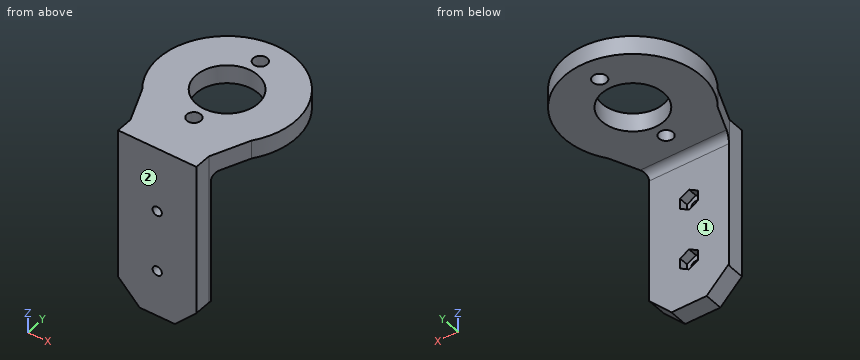
Autodesk Inventor part; units mm, degrees
ref_plane "YZ Plane" through (0, 0, 0) normal (1, 0, 0) x (0, 1, 0)
ref_plane "XZ Plane" through (0, 0, 0) normal (0, 1, 0) x (-1, 0, 0)
ref_plane "XY Plane" through (0, 0, 0) normal (0, 0, 1) x (1, 0, 0)
sketch "Sketch1" plane through (0, 0, 0) normal (0, 0, 1) x (1, 0, 0)
  circle A0 centre (0, 0) radius 22.1
  circle A1 centre (0, 14.5) radius 2.25
  circle A2 centre (0, -14.5) radius 2.25
  line L0 (0, 14.5) -> (0, -14.5)
  circle A3 centre (0, 0) radius 10
  line L1 (-12.7, -18.086459) -> (-12.7, -30.5)
  line L2 (-12.7, -30.5) -> (12.7, -30.5)
  line L3 (12.7, -30.5) -> (12.7, -18.086459)
  line L4 (-12.7, -24.5) -> (12.7, -24.5)
  point P0 (0, -30.5)
  dimension "d0" = 44.2
  dimension "d1" = 29
  dimension "d2" = 4.5
  dimension "d3" = 20
  dimension "d4" = 30.5
  dimension "d5" = 6
  dimension "d23" = 25.4
sketch "Sketch1 outline for Extrusion1" plane through (0, 0, 0) normal (0, 0, 1) x (1, 0, 0)
  arc A0 (12.7, -18.086459) -> (-12.7, -18.086459) centre (0, 0) ccw
  line L0 (12.7, -30.5) -> (12.7, -18.086459)
  line L1 (-12.7, -18.086459) -> (-12.7, -30.5)
  line L2 (-12.7, -30.5) -> (12.7, -30.5)
  circle A1 centre (0, -14.5) radius 2.25
  circle A2 centre (0, 14.5) radius 2.25
  circle A3 centre (0, 0) radius 10
extrude "Extrusion1" add sketch "Sketch1 outline for Extrusion1" along normal blind 6
sketch "Sketch1 outline for Extrusion2" plane through (0, 0, 0) normal (0, 0, 1) x (1, 0, 0)
  line L0 (-12.7, -30.5) -> (12.7, -30.5)
  line L1 (-12.7, -24.5) -> (-12.7, -30.5)
  line L2 (12.7, -24.5) -> (-12.7, -24.5)
  line L3 (12.7, -30.5) -> (12.7, -24.5)
extrude "Extrusion2" add sketch "Sketch1 outline for Extrusion2" against normal blind 50
fillet "Fillet1" radius 2.5 1 edges at (0, -24.5, 0)
sketch "Sketch2" plane through (-12.7, -30.5, 6) normal (0, -1, 0) x (1, 0, 0)
  circle A0 centre (12.7, -41) radius 1.5
  circle A1 centre (12.7, -21) radius 1.5
  line L0 (25.4, -56) -> (0, -56)
  point P0 (12.7, -6)
  point P1 (12.7, -56)
  dimension "d11" = 20
  dimension "d12" = 15
  dimension "d13" = 3
sketch "Sketch2 outline for Extrusion3" plane through (-12.7, -30.5, 6) normal (0, -1, 0) x (1, 0, 0)
  circle A0 centre (12.7, -21) radius 1.5
  circle A1 centre (12.7, -41) radius 1.5
extrude "Extrusion3" cut sketch "Sketch2 outline for Extrusion3" against normal blind 50
sketch "Sketch3" plane through (-12.7, -24.5, -50) normal (0, 1, 0) x (1, 0, 0)
  circle A0 centre (12.7, -35) radius 1.5
  circle A1 centre (12.7, -15) radius 1.5
  line L0 (25.4, -47.5) -> (0, -47.5)
  line L1 (25.4, -47.5) -> (25.4, 0)
  line L2 (0, 0) -> (25.4, 0)
  line L3 (0, -47.5) -> (0, 0)
  line L4 (12.7, -18.348632) -> (9.8, -16.674316)
  line L5 (9.8, -16.674316) -> (9.8, -13.325684)
  line L6 (9.8, -13.325684) -> (12.7, -11.651368)
  line L7 (12.7, -11.651368) -> (15.6, -13.325684)
  line L8 (15.6, -13.325684) -> (15.6, -16.674316)
  line L9 (15.6, -16.674316) -> (12.7, -18.348632)
  line L10 (12.7, -31.651368) -> (15.6, -33.325684)
  line L11 (15.6, -33.325684) -> (15.6, -36.674316)
  line L12 (15.6, -36.674316) -> (12.7, -38.348632)
  line L13 (12.7, -38.348632) -> (9.8, -36.674316)
  line L14 (9.8, -36.674316) -> (9.8, -33.325684)
  line L15 (9.8, -33.325684) -> (12.7, -31.651368)
  point P0 (12.7, -50)
  point P1 (12.7, -15)
  point P2 (12.7, -35)
  point P3 (15.6, -15)
  dimension "d16" = 5.8
  dimension "d17" = 5.8
sketch "Sketch3 outline for Extrusion4" plane through (-12.7, -24.5, -50) normal (0, 1, 0) x (1, 0, 0)
  line L0 (12.7, -18.348632) -> (15.6, -16.674316)
  line L1 (9.8, -16.674316) -> (12.7, -18.348632)
  line L2 (15.6, -16.674316) -> (15.6, -13.325684)
  line L3 (9.8, -13.325684) -> (9.8, -16.674316)
  line L4 (15.6, -13.325684) -> (12.7, -11.651368)
  line L5 (12.7, -11.651368) -> (9.8, -13.325684)
  circle A0 centre (12.7, -15) radius 1.5
  line L6 (12.7, -31.651368) -> (9.8, -33.325684)
  line L7 (15.6, -33.325684) -> (12.7, -31.651368)
  line L8 (9.8, -33.325684) -> (9.8, -36.674316)
  line L9 (15.6, -36.674316) -> (15.6, -33.325684)
  line L10 (9.8, -36.674316) -> (12.7, -38.348632)
  line L11 (12.7, -38.348632) -> (15.6, -36.674316)
  circle A1 centre (12.7, -35) radius 1.5
extrude "Extrusion4" cut sketch "Sketch3 outline for Extrusion4" against normal blind 3
chamfer "Chamfer1" distance 7 angle 45 2 edges at (12.7, -27.5, -50) (-12.7, -27.5, -50)
chamfer "Chamfer2" distance 7 angle 45 2 edges at (12.7, -18.0865, 3) (-12.7, -18.0865, 3)
properties part number "MOTOR_NUEVO_DC" material "Steel, Mild, Welded"
The model under review builds one solid part; all positions refer to its coordinate system, in mm. Face numbers are marked on the shaded views. A direction names the side the tool comes from. Give positions to 0.01 mm unless a question says otherwise; leave off trailing zeros. Order: outer loops, then holes, each group sorted by start corner. A loop starts at its lowest first (then second) coordinate and runs counter-clockwise, first axis right, second up. Notation, with made-up numbers: M -1.75,52 L 22.25,52 A22 ccw 22.25,75 Z; hole C -6,51.5 d11. An arc over 180 degrees is marked long. Use one line per item in the form item = value. Start each with the question number.
Item 1: We need section C-C on x = -8. Give the boundary of the cut face in (y, z), plus the area to 3 significant figures.
Item 2: Insertion check: pin 1 Ø5 at (x, z) = (1.5, -24) entering from +Y; pin 2 Ø5 at (x, z) = (0, -15) entering from +Y; pin 3 Ø3.5 at (y, z) = (-26, -15) entering from +X; pin 4 Ø6 at (x, y) = (-1, 4.5) entering from -Z. Each pin has a flat end and moves straight along its axis. Give the tip position at first contact, or say it passes through.
Item 3: For the marked faces 1 and 2, list the 3-axis set-ups (+Z, -Z, +X, -X, +Y, -Y) from which the entire face can be reached by the end or side of a thin tool; tool diameter is ignored.
Item 4: We need section D-D on z = -46. Give the boundary of the cut face in (x, y), plus the area to 3 significant figures.
Item 5: To check wall thickness, follow line 1 along Y through (x, z) = (0, 2); line 2 along X through (y, z) = (-29, -15); line 3 along Z through (x, y) = (0, -28). State the ranges of each line that lie inside material, in increasing order. Write a range as from..to.
Item 6: We need section B-B on y = 0. Give the boundary of the cut face in (x, z), plus the area to 3 significant figures.
Item 7: We need section A-A on z = -35. Give the boundary of the cut face in (x, y), plus the area to 3 significant figures.
Completed:
q1.outline = M -30.5,-47.7 L -24.5,-47.7 L -24.5,-2.5 A2.5 cw -22,0 L -6,0 L -6,6 L -30.5,6 Z; M 6,0 L 20.6,0 L 20.6,6 L 6,6 Z
q1.area = 522 mm²
q2.pin_1 = -24.5
q2.pin_2 = -27.5
q2.pin_3 = 12.95
q2.pin_4 = through
q3.face_1 = -Z, +X, -X, +Y
q3.face_2 = +Z, -Z, +X, -X, -Y
q4.outline = M -9.7,-30.5 L 9.7,-30.5 L 9.7,-24.5 L -9.7,-24.5 Z
q4.area = 116 mm²
q5.line_1 = -30.5..-16.75, -12.25..-10, 10..12.25, 16.75..22.1
q5.line_2 = -12.7..-1.5, 1.5..12.7
q5.line_3 = -50..-36.5, -33.5..-16.5, -13.5..6
q6.outline = M -22.1,0 L -10,0 L -10,6 L -22.1,6 Z; M 10,0 L 22.1,0 L 22.1,6 L 10,6 Z
q6.area = 145 mm²
q7.outline = M -12.95,-24.5 L -12.7,-25.09 L -12.7,-30.5 L -1.5,-30.5 L -1.5,-27.5 L -2.9,-27.5 L -2.9,-24.5 Z; M 1.5,-30.5 L 12.7,-30.5 L 12.7,-25.09 L 12.95,-24.5 L 2.9,-24.5 L 2.9,-27.5 L 1.5,-27.5 Z
q7.area = 126 mm²
